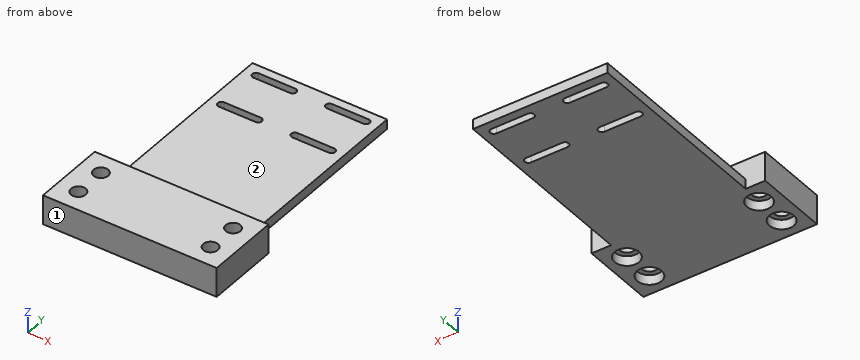
```python
from build123d import *

# Parameters (mm, degrees)
SKETCH1_W           = 55
SKETCH1_H           = 30
BOSS_EXTRUDE1_DEPTH = 4
SKETCH4_W           = 55
SKETCH4_H           = 4
BOSS_EXTRUDE2_DEPTH = 80
SKETCH5_W           = 4
SKETCH5_H           = 30
BOSS_EXTRUDE3_DEPTH = 8
SKETCH6_W           = 4
SKETCH6_H           = 30
BOSS_EXTRUDE4_DEPTH = 8
SKETCH7_W           = 71
SKETCH7_H           = 30
BOSS_EXTRUDE5_DEPTH = 8
SKETCH9_R           = 3
CUT_EXTRUDE1_DEPTH  = 8
SKETCH8_R           = 5
CUT_EXTRUDE4_DEPTH  = 4


with BuildPart() as part:
    # Sketch1 → Boss-Extrude1 (new body)
    with BuildSketch(Plane.XY):
        with Locations((0, 20)):
            Rectangle(SKETCH1_W, SKETCH1_H)
        with BuildLine():
            Line((22.5, 31.5), (7.5, 31.5))
            ThreePointArc((7.5, 31.5), (6, 30), (7.5, 28.5))
            Line((7.5, 28.5), (22.5, 28.5))
            ThreePointArc((22.5, 28.5), (24, 30), (22.5, 31.5))
        make_face(mode=Mode.SUBTRACT)
        with BuildLine():
            Line((22.5, 8.5), (7.5, 8.5))
            ThreePointArc((7.5, 8.5), (6, 10), (7.5, 11.5))
            Line((7.5, 11.5), (22.5, 11.5))
            ThreePointArc((22.5, 11.5), (24, 10), (22.5, 8.5))
        make_face(mode=Mode.SUBTRACT)
        with BuildLine():
            Line((-22.5, 8.5), (-7.5, 8.5))
            ThreePointArc((-7.5, 8.5), (-6, 10), (-7.5, 11.5))
            Line((-7.5, 11.5), (-22.5, 11.5))
            ThreePointArc((-22.5, 11.5), (-24, 10), (-22.5, 8.5))
        make_face(mode=Mode.SUBTRACT)
        with BuildLine():
            Line((-7.5, 28.5), (-22.5, 28.5))
            ThreePointArc((-22.5, 28.5), (-24, 30), (-22.5, 31.5))
            Line((-22.5, 31.5), (-7.5, 31.5))
            ThreePointArc((-7.5, 31.5), (-6, 30), (-7.5, 28.5))
        make_face(mode=Mode.SUBTRACT)
    extrude(amount=BOSS_EXTRUDE1_DEPTH)

    # Sketch4 → Boss-Extrude2 (add)
    with BuildSketch(Plane.XZ.offset(-5)):
        with Locations((0, 2)):
            Rectangle(SKETCH4_W, SKETCH4_H)
    extrude(amount=BOSS_EXTRUDE2_DEPTH)

    # Sketch5 → Boss-Extrude3 (add)
    with BuildSketch(Plane.ZY.offset(27.5)):
        with Locations((2, -60)):
            Rectangle(SKETCH5_W, SKETCH5_H)
    extrude(amount=BOSS_EXTRUDE3_DEPTH)

    # Sketch6 → Boss-Extrude4 (add)
    with BuildSketch(Plane(origin=(27.5, 0, 0), x_dir=(0, 0, -1), z_dir=(1, 0, 0))):
        with Locations((-2, -60)):
            Rectangle(SKETCH6_W, SKETCH6_H)
    extrude(amount=BOSS_EXTRUDE4_DEPTH)

    # Sketch7 → Boss-Extrude5 (add)
    with BuildSketch(Plane.XY.offset(4)):
        with Locations((0, -60)):
            Rectangle(SKETCH7_W, SKETCH7_H)
    extrude(amount=BOSS_EXTRUDE5_DEPTH)

    # Sketch9 → Cut-Extrude1 (cut)
    with BuildSketch(Plane.XY.offset(12)):
        with Locations((27.014718626, -66.514718626)):
            Circle(SKETCH9_R)
        with Locations((27.014718626, -53.485281374)):
            Circle(SKETCH9_R)
        with Locations((-27.014718626, -53.485281374)):
            Circle(SKETCH9_R)
        with Locations((-27.014718626, -66.514718626)):
            Circle(SKETCH9_R)
    extrude(amount=-CUT_EXTRUDE1_DEPTH, mode=Mode.SUBTRACT)

    # Sketch8 → Cut-Extrude4 (cut)
    with BuildSketch(Plane(origin=(0, 0, 0), x_dir=(-1, 0, 0), z_dir=(0, 0, -1))):
        with Locations((-27.014718626, -53.485281374)):
            Circle(SKETCH8_R)
        with Locations((-27.014718626, -66.514718626)):
            Circle(SKETCH8_R)
        with Locations((27.014718626, -53.485281374)):
            Circle(SKETCH8_R)
        with Locations((27.014718626, -66.514718626)):
            Circle(SKETCH8_R)
    extrude(amount=-CUT_EXTRUDE4_DEPTH, mode=Mode.SUBTRACT)


solid = part.part
```
Geometry check sheet. Reference: the model listing, model coordinates, mm. Face numbers are marked on the shaded views. A direction names the side the tool comes from. Round coordinates to 2 decimals unless told otherwise and drop trailing zeros. Loops run counter-clockwise (first coordinate to the right, second up) from the corner with the lowest first, then second, coordinate; pieces in that order, holes last. Notation, with made-up numbers: M -27,-1 L 26,-1 A21 ccw 26,17 Z; hole C 48,-13.5 d6. An arc over 180 degrees is marked long. Return JSON: item names as keys, results as strings. Group by question number.
(1) Go/stop test with flat-tipped pins: pin 1 (3.5 mm diameter, centred on x = 27.01, y = -66.51, fed in from -Z); pin 2 (1.5 mm diameter, centred on y = 0.5, z = 1.5, fed in from -X); pin 3 (8 mm diameter, centred on x = 28.5, y = -66.5, fed in from -Z); pin 4 (9.5 mm diameter, centred on x = 27.01, y = -53.49, fed in from -Z). Record where each tip stops, or that it passes through.
(2) Section check A-A, the plane y = 10. Enter the section's corners in (x, z).
(3) Section check D-D, the plane x = 0. Enter the section's corners in (y, z), and give its area (3 significant figures).
(4) Set-up check for the marked faces 1 and 2: record each of +Z, -Z, +X, -X, +Y, -Y from which the full face is reachable in a straight line by a thin tool's end or side.
(5) Scan lines: line 1 along Y through (x, z) = (16.5, 3.5); line 2 along Y through (x, z) = (-29, 5.5); line 3 along X through (y, z) = (-55, 9.75). Record each from-to range of solid material in increasing order. Write a range as [from, to].
(6) Section check B-B, the plane x = -16. Enter the section's corners in (y, z).
(7) Section check C-C, the plane z = 5.5. Enter the section's corners in (x, y), and give its area (3 significant figures).
Data:
{
 "1": {"pin 1": "through", "pin 2": "x = -27.5", "pin 3": "z = 0", "pin 4": "z = 4"},
 "2": {"outline": "M -27.5,0 L -24,0 L -24,4 L -27.5,4 Z; M -6,0 L 6,0 L 6,4 L -6,4 Z; M 24,0 L 27.5,0 L 27.5,4 L 24,4 Z"},
 "3": {"outline": "M -75,0 L 35,0 L 35,4 L -45,4 L -45,12 L -75,12 Z", "area": "680 mm²"},
 "4": {"face 1": "+Z, -Z, +X, -X, -Y", "face 2": "+Z, +X, -X, +Y"},
 "5": {"line 1": "[-75, 8.5], [11.5, 28.5], [31.5, 35]", "line 2": "[-75, -68.76], [-64.27, -55.73], [-51.24, -45]", "line 3": "[-35.5, -29.6], [-24.43, 24.43], [29.6, 35.5]"},
 "6": {"outline": "M -75,0 L 8.5,0 L 8.5,4 L -45,4 L -45,12 L -75,12 Z; M 11.5,0 L 28.5,0 L 28.5,4 L 11.5,4 Z; M 31.5,0 L 35,0 L 35,4 L 31.5,4 Z"},
 "7": {"outline": "M -35.5,-75 L 35.5,-75 L 35.5,-45 L -35.5,-45 Z; hole C -27.01,-66.51 d6; hole C -27.01,-53.49 d6; hole C 27.01,-66.51 d6; hole C 27.01,-53.49 d6", "area": "2,020 mm²"}
}
